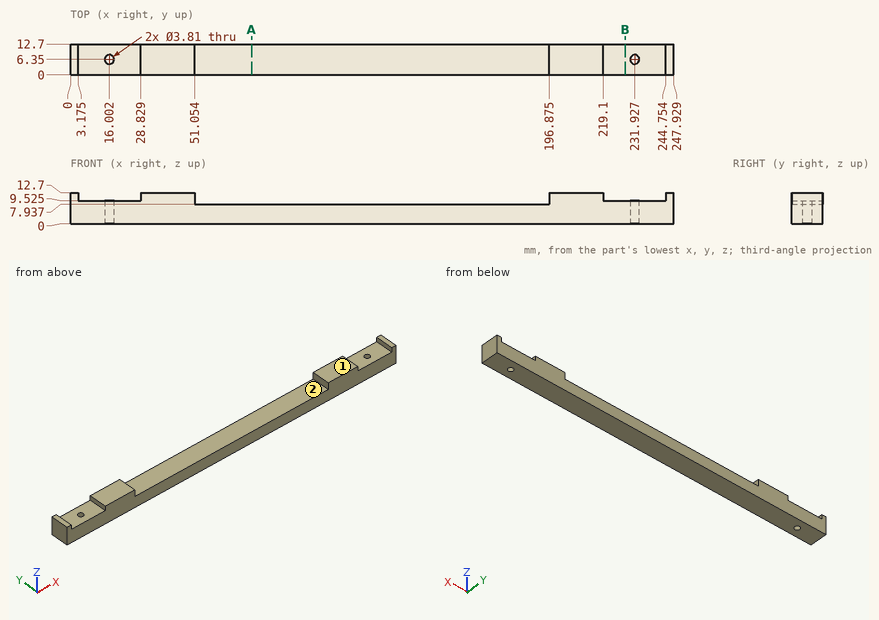
Here's the drawing with two shaded views (mm, measured from the low corner). I have some questions. Give positions to 0.01 mm unless a question says otherwise; leave off trailing zeros. Write each loop counter-clockwise with the first axis right and the second up, starting at its lowest first coordinate (ties: lowest second). Pieces come first, ordered by that corner, then holes. Notation, with made-up numbers: (-2.75, -25.5) - (56.25, -25.5) arc R12 ccw to (56.25, -20.5) - close; hole circle Ø6 at (45, -14.5). An arc over 180 degrees is marked (long way). One line per item, written item: value. Start each with the question number.
Item 1: Please list where these lines run through material, in increasing order: line 1 (X direction, y = 6.25, z = 5.25) (1 decimal); line 2 (X direction, y = 7.5, z = 10.75) (1 decimal); line 3 (X direction, y = 7.5, z = 5) (1 decimal). Write a range as from..to.
Item 2: If we mould it in two halves opening along X, with no side actions, what happens to the marked faces 1 and 2? For each: +X half, -X half, draft (parallel to the pull), parting line (faces both ways), or undercut.
Item 3: Imagine slicing it at B-B, the plane x = 228. List the corners of the cut face in (y, z) for me (1 decimal), and give its area (3 significant figures).
Item 4: Imagine slicing it at A-A, the plane x = 74.5. List the corners of the cut face in (y, z) for me.
Item 5: I'm going to push flat-ended pins straight in: pin 1 (4 mm diameter, centred on x = 101.5, y = 5.5, fed in from +Z); pin 2 (4 mm diameter, centred on y = 9, z = 9.5, fed in from -X); pin 3 (2.5 mm diameter, centred on x = 231.93, y = 6.35, fed in from +Z); pin 4 (4 mm diameter, centred on x = 229.5, y = 3.5, fed in from +Z) (1 decimal). Where does each tip first touch, or does it pass through?
Geometry says:
1. line 1: 0..14.1, 17.9..230, 233.8..247.9
1. line 2: 0..3.2, 28.8..51.1, 196.9..219.1, 244.8..247.9
1. line 3: 0..14.5, 17.5..230.4, 233.4..247.9
2. face 1: draft
2. face 2: undercut
3. outline: (0, 0) - (12.7, 0) - (12.7, 9.5) - (0, 9.5) - close
3. area: 121 mm^2
4. outline: (0, 0) - (12.7, 0) - (12.7, 7.94) - (0, 7.94) - close
5. pin 1: z = 7.94
5. pin 2: x = 0
5. pin 3: through
5. pin 4: z = 9.5
